Autodesk Inventor part; units mm, degrees
ref_plane "YZ Plane" through (0, 0, 0) normal (1, 0, 0) x (0, 1, 0)
ref_plane "XZ Plane" through (0, 0, 0) normal (0, 1, 0) x (-1, 0, 0)
ref_plane "XY Plane" through (0, 0, 0) normal (0, 0, 1) x (1, 0, 0)
sketch "Sketch1" plane through (0, 0, 0) normal (0, 0, 1) x (1, 0, 0)
  line L0 (-22.5, 0) -> (22.5, 0)
  line L1 (22.5, 0) -> (22.5, 5)
  line L2 (-22.5, 0) -> (-22.5, 5)
  line L3 (-22.5, 5) -> (-9.5, 5)
  line L4 (22.5, 5) -> (9.5, 5)
  line L5 (-9.5, 5) -> (-9.5, 10)
  line L6 (9.5, 5) -> (9.5, 10)
  arc A0 (4, 18.6042) -> (-4, 18.6042) centre (0, 27) ccw
  line L7 (4, 18.6042) -> (8.9676, 10)
  line L8 (-4, 18.6042) -> (-8.9676, 10)
  line L9 (-9.5, 10) -> (9.5, 10) construction
  line L10 (-8.9676, 10) -> (-9.5, 10) construction
  line L11 (-8.9676, 10) -> (-9.5, 10)
  line L12 (8.9676, 10) -> (9.5, 10)
  line L13 (-11.4601, 5) -> (-11.4601, 0) construction
  line L14 (-16.9601, 5) -> (-16.9601, 0) construction
  line L15 (13.0399, 5) -> (13.0399, 0) construction
  line L16 (18.5399, 5) -> (18.5399, 0) construction
  arc A1 (-4, 18.6042) -> (4, 18.6042) centre (0, 27) ccw construction
  point P0 (0, 0)
  point P1 (0, 0)
  point P2 (0, 17.7)
  point P3 (15.7899, 5)
  point P4 (-14.2101, 5)
  dimension "B" = 45
  dimension "t" = 5
  dimension "d2" = 5
  dimension "dimensionf" = 19
  dimension "d4" = 13
  dimension "Y" = 10
  dimension "d6" = 5
  dimension "d" = 18.6
  dimension "e" = 22.5
  dimension "dimensionH" = 17.7
  dimension "dimensionh" = 27
  dimension "x" = 8
  dimension "d16" = 4
  dimension "dimensionc" = 30
  dimension "d21" = 6.7101
  dimension "s1" = 5.5
  dimension "d23" = 5.5
  dimension "d24" = 2.75
  dimension "d25" = 2.75
  dimension "d29" = 6
  dimension "d30" = 6
extrude "Extrusion1" add sketch "Sketch1" along normal blind 300
equation "\"d2\" = t"
properties part number "sbr20_300mm"
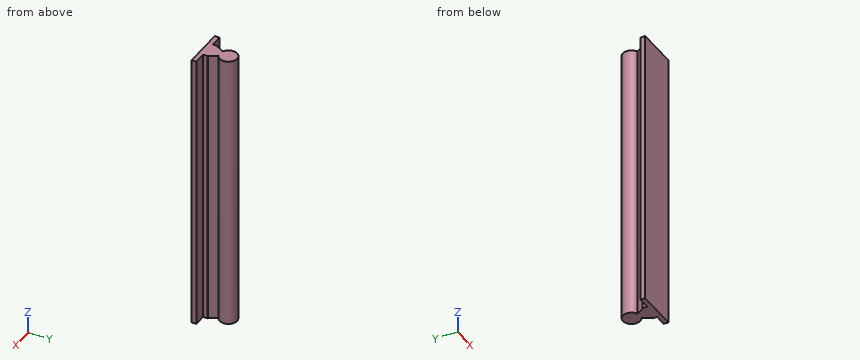
Could you check a few things on this model? Use its own coordinates, in mm. Round coordinates to 2 decimals unless told otherwise and drop trailing zeros. Write each loop counter-clockwise with the first axis right and the second up, starting at its lowest first coordinate (ties: lowest second). Pieces come first, ordered by that corner, then holes.
(1) For pin 1 (14.5 mm diameter, centred on x = 14, z = 121.5, fed in from +Y); pin 2 (4 mm diameter, centred on x = 1, z = 63.5, fed in from -Y); pin 3 (10 mm diameter, centred on y = 17, z = 100, fed in from -X); pin 4 (14.5 mm diameter, centred on x = -13.5, z = 141.5, fed in from +Y), each with a flat end and sliding along its axis, tell me the tip position at first contact or that it passes through.
Findings below:
pin 1: stops at y = 33.4
pin 2: stops at y = 0
pin 3: stops at x = -7.84
pin 4: stops at y = 33.89
(2) Suppose I cut it at C-C on y = 27. Write out the boundary of the cut face in (x, z).
Findings below:
outline: (-9.3, 0) - (9.3, 0) - (9.3, 300) - (-9.3, 300) - close
(3) Suppose I cut it at A-A on z = 68. Write out the boundary of the cut face in (x, y).
Findings below:
outline: (-22.5, 0) - (22.5, 0) - (22.5, 5) - (9.5, 5) - (9.5, 10) - (8.97, 10) - (4, 18.6) arc R9.3 ccw (long way) to (-4, 18.6) - (-8.97, 10) - (-9.5, 10) - (-9.5, 5) - (-22.5, 5) - close
(4) Suppose I cut it at B-B on x = 15.5. Write out the boundary of the cut face in (y, z), and give its area (3 significant figures).
Findings below:
outline: (0, 0) - (5, 0) - (5, 300) - (0, 300) - close
area: 1,500 mm2
(5) If I drill on probe 1 along Y at (x, z) = (12.5, 177); probe 2 along Y at (x, z) = (1, 190.5); probe 3 along Y at (x, z) = (-7.5, 87), over which ranges is the centre line in solid material (lowest first)?
Findings below:
probe 1: y = 0 to 5
probe 2: y = 0 to 36.25
probe 3: y = 0 to 12.54, 21.5 to 32.5
